```python
from build123d import *

# Parameters (mm, degrees)
F1_R          = 12.7
F1_R_2        = 11.1
F3_R          = 5.25
F4_DEPTH      = 12.7010001
F4_DEPTH_BACK = 12.7010001


with BuildPart() as f2:
    # F2: sweep along a path in F0
    with BuildLine(Plane.XY) as f2_path:
        ThreePointArc((1823.1628588801, -200), (1831.3636735329, -100.1494146961), (1834.1, 0))
    # F1 (on Front) → F2 (sweep)
    with BuildSketch(Plane.XZ):
        with Locations((1834.1, 0)):
            Circle(F1_R)
        with Locations((1834.1, 0)):
            Circle(F1_R_2, mode=Mode.SUBTRACT)
    sweep(path=f2_path.line)

    # F3 (on Top) → F4 (cut, two sides)
    with BuildSketch(Plane.XY) as f4_sk:
        with Locations((1833.6637668886, -40)):
            Circle(F3_R)
        with Locations((1827.1077718624, -160)):
            Circle(F3_R)
    extrude(amount=-F4_DEPTH, mode=Mode.SUBTRACT)
    extrude(f4_sk.sketch, amount=F4_DEPTH_BACK, mode=Mode.SUBTRACT)


solid = f2.part
```
Verification items for the finished model (mm, model axes). Coordinates: 2 decimals unless noted, no trailing zeros. Write each loop counter-clockwise with the first axis right and the second up, starting at its lowest first coordinate (ties: lowest second). Pieces come first, ordered by that corner, then holes. Notation, with made-up numbers: M 88,-23 L 131,-23 A4 cw 131,-16 Z; hole C -16.5,18 d9. An arc over 180 degrees is marked long. Answer as a JSON object with one key per item and string values. Group by question number.
(1) Gauge pin test, flat ends, axial feed: pin 1 (2 mm diameter, centred on x = 1820, y = -74.5, fed in from -Z); pin 2 (8.5 mm diameter, centred on x = 1827.11, y = -160, fed in from -Z); pin 3 (1 mm diameter, centred on y = -35.5, z = 9.5, fed in from +X); pin 4 (5 mm diameter, centred on x = 1829.5, z = 8.5, fed in from -Y). Record the tip position at first contact, or that the pin passes through.
(2) Release check for a two-part mould opening along X. For faces 1 (the face through (1833.22, 0, 11.23)), 2 (the face through (1828.42, -39.77, 11.22)), 3 (the face through (1822.287, -199.904, 11.23)), 4 (the face through (1828.42, -39.77, -11.22)) record: +X half, -X half, draft (parallel to the pull), parting line (faces both ways), or undercut.
(3) Cross-section at B-B, the plane x = 1825.5. State how many separate pieces and enclosed holes the cut face has, and give its area (3 significant figures).
(4) Cross-section at C-C, the plane z = -2. Record the cut outline in (x, y).
(5) Material ranges on line 1 (Z direction, x = 1832, y = -80); line 2 (X direction, y = -68.5, z = 5); line 3 (X direction, y = -69, z = 1.5), recorded low to high.
(6) Cross-section at A-A, the plane z = 7.25. Record the cut outline in (x, y), and give its area (3 significant figures).
Reply:
{
 "1": {"pin 1": "z = -5.22", "pin 2": "through", "pin 3": "x = 1842.72", "pin 4": "y = -200.97"},
 "2": {"face 1": "draft", "face 2": "undercut", "face 3": "-X half", "face 4": "undercut"},
 "3": {"separate pieces": "4", "enclosed holes": "0", "area": "728 mm²"},
 "4": {"outline": "M 1810.7,-198.63 L 1812.31,-198.81 A1823.18 ccw 1823.18,0 L 1821.56,0 A1821.56 cw Z; M 1834.02,-201.19 L 1835.63,-201.37 A1846.64 ccw 1846.64,0 L 1845.02,0 A1845.02 cw Z"},
 "5": {"line 1": "-12.7 to -11.09, 11.09 to 12.7", "line 2": "1821.14 to 1822.9, 1842.74 to 1844.5", "line 3": "1820.18 to 1821.8, 1843.81 to 1845.42"},
 "6": {"outline": "M 1812.8,-198.86 L 1814.81,-199.08 A1825.69 ccw 1825.69,0 L 1823.67,0 A1823.67 cw Z; M 1831.52,-200.92 L 1833.53,-201.14 A1844.53 ccw 1844.53,0 L 1842.51,0 A1842.51 cw Z", "area": "810 mm²"}
}
